Work out the finished part from the listing and answer in its coordinate system (mm). A direction names the side the tool comes from. Coordinates: 2 decimals unless noted, no trailing zeros. Write each loop counter-clockwise with the first axis right and the second up, starting at its lowest first coordinate (ties: lowest second). Pieces come first, ordered by that corner, then holes. Notation, with made-up numbers: (62, 81.5) - (101, 81.5) arc R31 cw to (101, 119.5) - close; hole circle Ø8 at (6.5, 75). An arc over 180 degrees is marked (long way). Use CSV: the item, a comma, the result in double quotes. Start each with the question number.
from build123d import *

# Parameters (mm, degrees)
SKETCH1_R          = 10
EXTRUDE1_DEPTH     = 25.4
CUT_EXTRUDE1_DEPTH = 26.4
CUT_EXTRUDE2_REACH = 122
SKETCH5_R          = 6
CUT_EXTRUDE3_REACH = 151
SKETCH6_R          = 1.5
SKETCH7_W          = 131.09029237
SKETCH7_H          = 20
EXTRUDE2_DEPTH     = 5
SKETCH8_R          = 15.5
SKETCH8_R_2        = 10
EXTRUDE3_DEPTH     = 3


with BuildPart() as part:
    # Sketch1 → Extrude1 (new body)
    with BuildSketch(Plane.XY):
        with BuildLine():
            Line((-38, 0), (38, 0))
            Line((38, 0), (38, -12))
            Line((38, -12), (45, -12))
            Line((45, -12), (45, 34.839604128))
            Line((45, 34.839604128), (18.793852416, 106.840402867))
            ThreePointArc((18.793852416, 106.840402867), (0, 120), (-18.793852416, 106.840402867))
            Line((-18.793852416, 106.840402867), (-45, 34.839604128))
            Line((-45, 34.839604128), (-45, -12))
            Line((-45, -12), (-38, -12))
            Line((-38, -12), (-38, 0))
        make_face()
        with Locations((0, 100)):
            Circle(SKETCH1_R, mode=Mode.SUBTRACT)
    extrude(amount=EXTRUDE1_DEPTH)

    # Sketch2 → Cut-Extrude1 (cut, through all)
    with BuildSketch(Plane.XY.offset(25.4)):
        with BuildLine():
            Line((-32, 10), (32, 10))
            ThreePointArc((32, 10), (34.121320344, 10.878679656), (35, 13))
            Line((35, 13), (35, 37))
            ThreePointArc((35, 37), (34.121320344, 39.121320344), (32, 40))
            Line((32, 40), (-32, 40))
            ThreePointArc((-32, 40), (-34.121320344, 39.121320344), (-35, 37))
            Line((-35, 37), (-35, 13))
            ThreePointArc((-35, 13), (-34.121320344, 10.878679656), (-32, 10))
        make_face()
    extrude(amount=-CUT_EXTRUDE1_DEPTH, mode=Mode.SUBTRACT)

    # Sketch5 → Cut-Extrude2 (cut, up to next)
    with BuildSketch(Plane.XZ, mode=Mode.PRIVATE) as cut_extrude2_sk1:
        with Locations((13, 12.7)):
            Circle(SKETCH5_R)
    cut_extrude2_tool1 = extrude(cut_extrude2_sk1.sketch, amount=-CUT_EXTRUDE2_REACH, mode=Mode.PRIVATE) & part.part
    add(cut_extrude2_tool1.solids().sort_by_distance((13, 0, 12.7))[0], mode=Mode.SUBTRACT)
    # Sketch5 → Cut-Extrude2 (cut, up to next)
    with BuildSketch(Plane.XZ, mode=Mode.PRIVATE) as cut_extrude2_sk2:
        with Locations((-17, 12.7)):
            Circle(SKETCH5_R)
    cut_extrude2_tool2 = extrude(cut_extrude2_sk2.sketch, amount=-CUT_EXTRUDE2_REACH, mode=Mode.PRIVATE) & part.part
    add(cut_extrude2_tool2.solids().sort_by_distance((-17, 0, 12.7))[0], mode=Mode.SUBTRACT)

    # Sketch6 → Cut-Extrude3 (cut, up to next)
    with BuildSketch(Plane(origin=(0, 137, 0), x_dir=(-1, 0, 0), z_dir=(0, 1, 0)), mode=Mode.PRIVATE) as cut_extrude3_sk1:
        with Locations((0, 12.7)):
            Circle(SKETCH6_R)
    cut_extrude3_tool1 = extrude(cut_extrude3_sk1.sketch, amount=-CUT_EXTRUDE3_REACH, mode=Mode.PRIVATE) & part.part
    add(cut_extrude3_tool1.solids().sort_by_distance((0, 137, 12.7))[0], mode=Mode.SUBTRACT)

    # Sketch7 → Extrude2 (cut)
    with BuildSketch(Plane.XY.offset(25.4)):
        with Locations((2.300736004, 68)):
            Rectangle(SKETCH7_W, SKETCH7_H)
    extrude(amount=-EXTRUDE2_DEPTH, mode=Mode.SUBTRACT)

    # Sketch8 → Extrude3 (cut)
    with BuildSketch(Plane.XY.offset(25.4)):
        with Locations((0, 100)):
            Circle(SKETCH8_R)
        with Locations((0, 100)):
            Circle(SKETCH8_R_2, mode=Mode.SUBTRACT)
    extrude3 = extrude(amount=-EXTRUDE3_DEPTH, mode=Mode.SUBTRACT)

    # Mirror1: Extrude3 across plane
    add(extrude3.mirror(Plane.XY.offset(12.7)), mode=Mode.SUBTRACT)


solid = part.part
Item 1: Straight lines are drawn through the part: probe 1 along Y at (x, z) = (0, 7.25); probe 2 along X at (y, z) = (-5, 22.25); probe 3 along X at (y, z) = (20, 11.25). For each, find the intervals that lie inside material, in ascending order. Write a range as [from, to].
Item 2: A cutting plane is placed at C-C (x = 21). Determine the outline of the cut face in (y, z), then the cut area to 3 significant figures.
Item 3: Each of these flat-tipped pins is pushed along its axis until it touches: pin 1 (9.5 mm diameter, centred on x = -3.5, y = 92.5, fed in from -Z); pin 2 (8 mm diameter, centred on x = -14.5, z = 16.5, fed in from +Y); pin 3 (8 mm diameter, centred on y = 83.5, z = 9, fed in from +X); pin 4 (22 mm diameter, centred on x = 6.5, y = 65.5, fed in from +Z). Where does it stop, or does it pass through?
Item 4: A cutting plane is placed at A-A (x = 5.5). Determine the outline of the cut face in (y, z), then the cut area to 3 significant figures.
Item 5: A cutting plane is placed at B-B (y = 100). Determine the outline of the cut face in (x, z).
Item 6: Which of the six approach directions +Z, -Z, +X, -X, +Y, -Y give full straight-line access (tool end or side, diameter ignored) to faces 5 (the face through (34.14, 39.1, 12.88)), 6 (the face through (38, -6, 13)), 7 (the face through (0.325, 115.013, 11.236)), 8 (the face through (3, 90, 22.4))?
Item 7: Determine the mould class of faces 1 (the face through (-1, 8, 25.4)), 2 (the face through (0, 10, 13)), 3 (the face through (-45, 12, 13)), 4 (the face through (-2.018, 115.368, 1.479)) for opening direction X: +X half, -X half, draft (parallel to the pull), parting line (faces both ways), or undercut.
Calculated:
1,probe 1,"y = [0, 10], [40, 90], [110, 120]"
1,probe 2,"x = [-45, -38], [38, 45]"
1,probe 3,"x = [-45, -35], [35, 45]"
2,outline,"(0, 0) - (10, 0) - (10, 25.4) - (0, 25.4) - close; (40, 0) - (100.78, 0) - (100.78, 25.4) - (78, 25.4) - (78, 20.4) - (58, 20.4) - (58, 25.4) - (40, 25.4) - close"
2,area,"1,700 mm²"
3,pin 1,"stops at z = 3"
3,pin 2,"stops at y = 117.02"
3,pin 3,"stops at x = 28.74"
3,pin 4,"stops at z = 25.4"
4,outline,"(0, 0) - (10, 0) - (10, 25.4) - (0, 25.4) - close; (40, 0) - (85.51, 0) - (85.51, 3) - (91.65, 3) - (91.65, 22.4) - (85.51, 22.4) - (85.51, 25.4) - (78, 25.4) - (78, 20.4) - (58, 20.4) - (58, 25.4) - (40, 25.4) - close; (108.35, 3) - (114.49, 3) - (114.49, 0) - (119.23, 0) - (119.23, 25.4) - (114.49, 25.4) - (114.49, 22.4) - (108.35, 22.4) - close"
4,area,"1,670 mm²"
5,outline,"(-21.28, 0) - (-15.5, 0) - (-15.5, 3) - (-10, 3) - (-10, 22.4) - (-15.5, 22.4) - (-15.5, 25.4) - (-21.28, 25.4) - close; (10, 3) - (15.5, 3) - (15.5, 0) - (21.28, 0) - (21.28, 25.4) - (15.5, 25.4) - (15.5, 22.4) - (10, 22.4) - close"
6,face 5,"+Z, -Z"
6,face 6,"+Z, -Z, -Y"
6,face 7,"+Y"
6,face 8,"+Z"
7,face 1,"draft"
7,face 2,"undercut"
7,face 3,"-X half"
7,face 4,"undercut"
